from build123d import *

# Parameters (mm, degrees)
SKETCH4_W                = 12.46
SKETCH4_H                = 17.25
BOSS_EXTRUDE3_DEPTH      = 6
SKETCH8_R                = 12.546781182
SKETCH8_R_2              = 11.15
BOSS_EXTRUDE6_DEPTH      = 8.3
BOSS_EXTRUDE6_DEPTH_BACK = 17.25
BOSS_EXTRUDE4_DEPTH      = 17.25
SKETCH6_R                = 0.75
CUT_EXTRUDE1_DEPTH       = 5
CHAMFER1_SIZE            = 0.5
CHAMFER1_SIZE2           = 0.866025404
SKETCH10_W               = 12.46
SKETCH10_H               = 23.7
CUT_EXTRUDE3_DEPTH       = 17.25
BOSS_EXTRUDE7_DEPTH      = 8.3
BOSS_EXTRUDE9_DEPTH      = 10
SKETCH20_R               = 11.15
SKETCH20_R_2             = 7.15
BOSS_EXTRUDE11_DEPTH     = 8.3
SKETCH21_R               = 10.15
SKETCH21_R_2             = 7.15
CUT_EXTRUDE7_DEPTH       = 1.3
SKETCH11_W               = 10
SKETCH11_H               = 2
CUT_EXTRUDE4_DEPTH       = 23.7
CUT_EXTRUDE8_REACH       = 37.55
SKETCH24_W               = 12.46
SKETCH24_H               = 6
BOSS_EXTRUDE10_DEPTH     = 25.093562
SKETCH18_W               = 21.5
SKETCH18_H               = 12.438292938
CUT_EXTRUDE5_DEPTH       = 2
SKETCH19_R               = 3.5
CUT_EXTRUDE6_DEPTH       = 43.5
CUT_EXTRUDE6_DEPTH_BACK  = 3
FILLET1_R                = 7
SKETCH22_R               = 6.5
BOSS_EXTRUDE12_DEPTH     = 5
SKETCH23_R               = 6.075
BOSS_EXTRUDE13_DEPTH     = 5
FILLET2_R                = 1
BOSS_EXTRUDE15_DEPTH     = 2
CUT_EXTRUDE9_REACH       = 46.5
SKETCH26_R               = 0.75


with BuildPart() as part:
    # Sketch4 → Boss-Extrude3 (new body)
    with BuildSketch(Plane.XY):
        with Locations((0, -1.35)):
            Rectangle(SKETCH4_W, SKETCH4_H)
    extrude(amount=BOSS_EXTRUDE3_DEPTH)



with BuildPart() as body_2:
    # Sketch8 → Boss-Extrude6 (new body, two sides)
    with BuildSketch(Plane(origin=(0, -9.975, 0), x_dir=(-1, 0, 0), z_dir=(0, -1, 0))) as boss_extrude6_sk:
        with Locations((0, -23.55)):
            Circle(SKETCH8_R)
        with Locations((0, -23.55)):
            Circle(SKETCH8_R_2, mode=Mode.SUBTRACT)
    extrude(amount=BOSS_EXTRUDE6_DEPTH)
    extrude(boss_extrude6_sk.sketch, amount=-BOSS_EXTRUDE6_DEPTH_BACK)


with BuildPart() as part_1:
    add(part.part)

    add(body_2.part)  # Boss-Extrude4 merges body 2
    # Sketch5 → Boss-Extrude4 (add)
    with BuildSketch(Plane(origin=(0, 7.275, 0), x_dir=(1, 0, 0), z_dir=(0, 1, 0))):
        with BuildLine():
            Line((12.546781182, -23.55), (12.546781182, 0))
            Line((12.546781182, 0), (6.23, 0))
            Line((6.23, 0), (6.23, -29.7))
            Line((6.23, -29.7), (-6.23, -29.7))
            Line((-6.23, -29.7), (-6.23, 0))
            Line((-6.23, 0), (-12.546781182, 0))
            Line((-12.546781182, 0), (-12.546781182, -23.55))
            ThreePointArc((-12.546781182, -23.55), (0, -36.096781182), (12.546781182, -23.55))
        make_face()
    extrude(amount=-BOSS_EXTRUDE4_DEPTH)

    # Sketch6 → Cut-Extrude1 (cut)
    with BuildSketch(Plane(origin=(0, 7.275, 0), x_dir=(1, 0, 0), z_dir=(0, 1, 0))):
        with Locations((0, -3.6)):
            Circle(SKETCH6_R)
        with Locations((0, -32.1)):
            Circle(SKETCH6_R)
    extrude(amount=-CUT_EXTRUDE1_DEPTH, mode=Mode.SUBTRACT)

    # Chamfer1
    chamfer1_edges = [part_1.edges().sort_by_distance(p)[0] for p in [
        (-0.75, 7.275, 3.6),
        (-0.75, 7.275, 32.1),
    ]]
    chamfer1_side = [part_1.faces().sort_by_distance(p)[0] for p in [
        (0, 7.275, 35.657160381),
    ]]
    chamfer(chamfer1_edges, length=CHAMFER1_SIZE, length2=CHAMFER1_SIZE2, reference=chamfer1_side[0])

    # Sketch10 → Cut-Extrude3 (cut)
    with BuildSketch(Plane(origin=(0, 7.275, 0), x_dir=(1, 0, 0), z_dir=(0, 1, 0))):
        with Locations((0, -17.85)):
            Rectangle(SKETCH10_W, SKETCH10_H)
    extrude(amount=-CUT_EXTRUDE3_DEPTH, mode=Mode.SUBTRACT)

    # Sketch13 → Boss-Extrude7 (add)
    with BuildSketch(Plane.XZ.offset(18.275)):
        with BuildLine():
            Line((-12.546781182, 23.55), (-12.546781182, 0))
            Line((-12.546781182, 0), (12.546781182, 0))
            Line((12.546781182, 0), (12.546781182, 23.55))
            ThreePointArc((12.546781182, 23.55), (0, 11.003218818), (-12.546781182, 23.55))
        make_face()
    extrude(amount=-BOSS_EXTRUDE7_DEPTH)

    # Sketch15 → Boss-Extrude9 (add)
    with BuildSketch(Plane(origin=(0, 7.275, 0), x_dir=(1, 0, 0), z_dir=(0, 1, 0))):
        with BuildLine():
            Line((-12.546781182, 0), (12.546781182, 0))
            Line((12.546781182, 0), (12.546781182, -23.55))
            ThreePointArc((12.546781182, -23.55), (0, -36.096781182), (-12.546781182, -23.55))
            Line((-12.546781182, -23.55), (-12.546781182, 0))
        make_face()
        with BuildLine():
            Line((-6.23, -0.8), (6.23, -0.8))
            Line((6.23, -0.8), (6.23, -33))
            ThreePointArc((6.23, -33), (5.790660172, -34.060660172), (4.73, -34.5))
            Line((4.73, -34.5), (-4.73, -34.5))
            ThreePointArc((-4.73, -34.5), (-5.790660172, -34.060660172), (-6.23, -33))
            Line((-6.23, -33), (-6.23, -0.8))
        make_face(mode=Mode.SUBTRACT)
    extrude(amount=BOSS_EXTRUDE9_DEPTH)

    # Sketch20 → Boss-Extrude11 (add)
    with BuildSketch(Plane.XZ.offset(18.275)):
        with Locations((0, 23.55)):
            Circle(SKETCH20_R)
        with Locations((0, 23.55)):
            Circle(SKETCH20_R_2, mode=Mode.SUBTRACT)
    extrude(amount=-BOSS_EXTRUDE11_DEPTH)

    # Sketch21 → Cut-Extrude7 (cut)
    with BuildSketch(Plane.XZ.offset(18.275)):
        with Locations((0, 23.55)):
            Circle(SKETCH21_R)
        with Locations((0, 23.55)):
            Circle(SKETCH21_R_2, mode=Mode.SUBTRACT)
    extrude(amount=-CUT_EXTRUDE7_DEPTH, mode=Mode.SUBTRACT)

    # Sketch11 → Cut-Extrude4 (cut)
    with BuildSketch(Plane.XY.offset(29.7)):
        with Locations((0, -10.975)):
            Rectangle(SKETCH11_W, SKETCH11_H)
    extrude(amount=-CUT_EXTRUDE4_DEPTH, mode=Mode.SUBTRACT)

    # Sketch24 → Cut-Extrude8 (cut, up to next)
    with BuildSketch(Plane.XZ.offset(18.275), mode=Mode.PRIVATE) as cut_extrude8_sk1:
        with Locations((0, 9)):
            Rectangle(SKETCH24_W, SKETCH24_H)
    cut_extrude8_tool1 = extrude(cut_extrude8_sk1.sketch, amount=-CUT_EXTRUDE8_REACH, mode=Mode.PRIVATE) & part_1.part
    add(cut_extrude8_tool1.solids().sort_by_distance((0, -18.275, 9))[0], mode=Mode.SUBTRACT)

    # Sketch17 → Boss-Extrude10 (add)
    with BuildSketch(Plane(origin=(-12.546781182, 4.728218818, 0), x_dir=(0, -1, 0), z_dir=(1, 0, 0))):
        Polygon((26.978218818, 26.5), (26.978218818, 0), (-17.521781182, 0), (-17.521781182, 26.5), (-13.521781182, 26.5), (-13.521781182, 5), (22.978218818, 5), (22.978218818, 26.5), align=None)
    extrude(amount=BOSS_EXTRUDE10_DEPTH)

    # Sketch18 → Cut-Extrude5 (cut)
    with BuildSketch(Plane.ZX.offset(-18.25)):
        with Locations((-15.75, 0)):
            Rectangle(SKETCH18_W, SKETCH18_H)
    extrude(amount=-CUT_EXTRUDE5_DEPTH, mode=Mode.SUBTRACT)

    # Sketch19 → Cut-Extrude6 (cut, two sides)
    with BuildSketch(Plane.ZX.offset(-20.25)) as cut_extrude6_sk:
        with Locations((-20, 0)):
            Circle(SKETCH19_R)
    extrude(amount=CUT_EXTRUDE6_DEPTH, mode=Mode.SUBTRACT)
    extrude(cut_extrude6_sk.sketch, amount=-CUT_EXTRUDE6_DEPTH_BACK, mode=Mode.SUBTRACT)

    # Fillet1
    fillet1_edges = [part_1.edges().sort_by_distance(p)[0] for p in [
        (12.546780818, -20.25, -26.5),
        (-12.546781182, -20.25, -26.5),
        (12.546780818, 20.25, -26.5),
        (-12.546781182, 20.25, -26.5),
    ]]
    fillet(fillet1_edges, radius=FILLET1_R)

    # Sketch22 → Boss-Extrude12 (add)
    with BuildSketch(Plane(origin=(0, 22.25, 0), x_dir=(1, 0, 0), z_dir=(0, 1, 0))):
        with Locations((0, 20)):
            Circle(SKETCH22_R)
    extrude(amount=-BOSS_EXTRUDE12_DEPTH)

    # Sketch23 → Boss-Extrude13 (add)
    with BuildSketch(Plane.XZ.offset(-17.25)):
        with Locations((0, -20)):
            Circle(SKETCH23_R)
    extrude(amount=BOSS_EXTRUDE13_DEPTH)

    # Fillet2
    fillet2_edges = [part_1.edges().sort_by_distance(p)[0] for p in [
        (-6.075, 12.25, -20),
    ]]
    fillet(fillet2_edges, radius=FILLET2_R)

    # Sketch25 → Boss-Extrude15 (add)
    with BuildSketch(Plane(origin=(0, -20.25, 0), x_dir=(1, 0, 0), z_dir=(0, 1, 0))):
        Polygon((-6.219146469, 5), (-2.5, 5), (-3.1585, 20), (-3.44385, 26.5), (-6.219146469, 26.5), align=None)
        Polygon((6.219146469, 5), (2.5, 5), (3.1585, 20), (3.44385, 26.5), (6.219146469, 26.5), align=None)
    extrude(amount=BOSS_EXTRUDE15_DEPTH)

    # Sketch26 → Cut-Extrude9 (cut, up to next)
    with BuildSketch(Plane(origin=(0, -22.25, 0), x_dir=(-1, 0, 0), z_dir=(0, -1, 0)), mode=Mode.PRIVATE) as cut_extrude9_sk1:
        with Locations((0, 10)):
            Circle(SKETCH26_R)
    cut_extrude9_tool1 = extrude(cut_extrude9_sk1.sketch, amount=-CUT_EXTRUDE9_REACH, mode=Mode.PRIVATE) & part_1.part
    add(cut_extrude9_tool1.solids().sort_by_distance((0, -22.25, -10))[0], mode=Mode.SUBTRACT)


solid = part_1.part
The listing builds one solid part. Answer for the finished solid, in the listing's coordinates (mm). A direction names the side the tool comes from. Round coordinates to 2 decimals unless told otherwise and drop trailing zeros. Write each loop counter-clockwise with the first axis right and the second up, starting at its lowest first coordinate (ties: lowest second). Pieces come first, ordered by that corner, then holes. Notation, with made-up numbers: (-23.75, 16.5) - (3.25, 16.5) arc R28 ccw to (3.25, 39.5) - close; hole circle Ø6 at (67.25, 86). An arc over 180 degrees is marked (long way). Use a Markdown table: item, result. Add a question column.
1. Consider line 1 (Z direction, x = 0, y = -13.5); line 2 (Z direction, x = 0, y = 5.2); line 3 (Z direction, x = 0, y = -18). Determine where each line is inside the solid, lowest interval first.
2. The part is cut by section B-B (z = 28). Write down the section's boundary in (x, y) (1 decimal), and give its area (3 significant figures).
3. A tool of negligible diameter and unlimited length cuts with its end or side. For faces 1 (the face through (-8, -18.25, -16)), 2 (the face through (6, -9.975, 29)), 3 (the face through (5, -18.275, 14)), 4 (the face through (-7, -16.975, 21)), from which of +Z, -Z, +X, -X, +Y, -Y can it reach the whole face along a straight path? Write none if from no direction.
4. The part is cut by section D-D (z = 3.6). Write down the section's boundary in (x, y) (3 decimals), and give its area (3 significant figures).
5. For a pull along Z with two mould halves and no side action, classify faces 5 (the face through (-0.098, 4.371, 2.856)), 6 (the face through (0, 2.275, 32)), 7 (the face through (8, -18.25, -16)), 8 (the face through (0, 20, 0)) as +Z half, -Z half, draft (parallel to the pull), parting line (faces both ways), or undercut.
6. Flat-ended cylindrical pins translate along their axes: P1, Ø5, axis at x = 3, y = -8.5, coming from the +Z side; P2, Ø0.6, axis at x = 5.5, z = 28.5, coming from the +Y side (3 decimals); P3, Ø1.5, axis at x = -8, y = 0.5, coming from the -Z side; P4, Ø12, axis at y = -7, z = -18.5, coming from the +X side. Find the tip coordinate at first contact, or state that the pin passes through.
7. The part is cut by section C-C (y = -14). Write down the section's boundary in (x, z).
8. The part is cut by section A-A (y = -2.5). Write down the section's boundary in (x, z).
Reported:
| question | item | result |
|---|---|---|
| 1 | line 1 | -5 to 6, 12 to 16.4, 30.7 to 36.1 |
| 1 | line 2 | -5 to 2.85, 4.35 to 6, 29.7 to 31.35, 32.85 to 36.1 |
| 1 | line 3 | -5 to 6, 12 to 13.4, 33.7 to 36.1 |
| 2 | outline | (-11.7, -18.3) - (-9.1, -18.3) - (-9.1, -17) - (-5.6, -17) - (-5.6, -10) - (-6.2, -10) - (-6.2, 17.3) - (-11.7, 17.3) - close; (5.6, -17) - (9.1, -17) - (9.1, -18.3) - (11.7, -18.3) - (11.7, 17.3) - (6.2, 17.3) - (6.2, -10) - (5.6, -10) - close |
| 2 | area | 392 mm^2 |
| 3 | face 1 | -Z, +X, -X |
| 3 | face 2 | +Y |
| 3 | face 3 | +Z, +X, -X, -Y |
| 3 | face 4 | -Y |
| 4 | outline | (-12.547, -18.275) - (12.547, -18.275) - (12.547, 17.275) - (6.23, 17.275) - (6.23, 7.275) - (1.25, 7.275) - (0.75, 6.409) - (0.75, 2.275) - (-0.75, 2.275) - (-0.75, 6.409) - (-1.25, 7.275) - (-6.23, 7.275) - (-6.23, 17.275) - (-12.547, 17.275) - close |
| 4 | area | 760 mm^2 |
| 5 | face 5 | undercut |
| 5 | face 6 | undercut |
| 5 | face 7 | draft |
| 5 | face 8 | +Z half |
| 6 | P1 | z = 36.09 |
| 6 | P2 | y = -9.975 |
| 6 | P3 | z = -5 |
| 6 | P4 | through |
| 7 | outline | (-12.55, -5) - (12.55, -5) - (12.55, 23.55) arc R12.55 ccw to (-12.55, 23.55) - close; hole circle Ø14.3 at (0, 23.55); hole (-6.23, 6) - (6.23, 6) - (6.23, 12) - (-6.23, 12) - close |
| 8 | outline | (-12.55, -5) - (12.55, -5) - (12.55, 23.55) arc R12.55 ccw to (-12.55, 23.55) - close; hole (-6.23, 6) - (6.23, 6) - (6.23, 29.7) - (-6.23, 29.7) - close |
